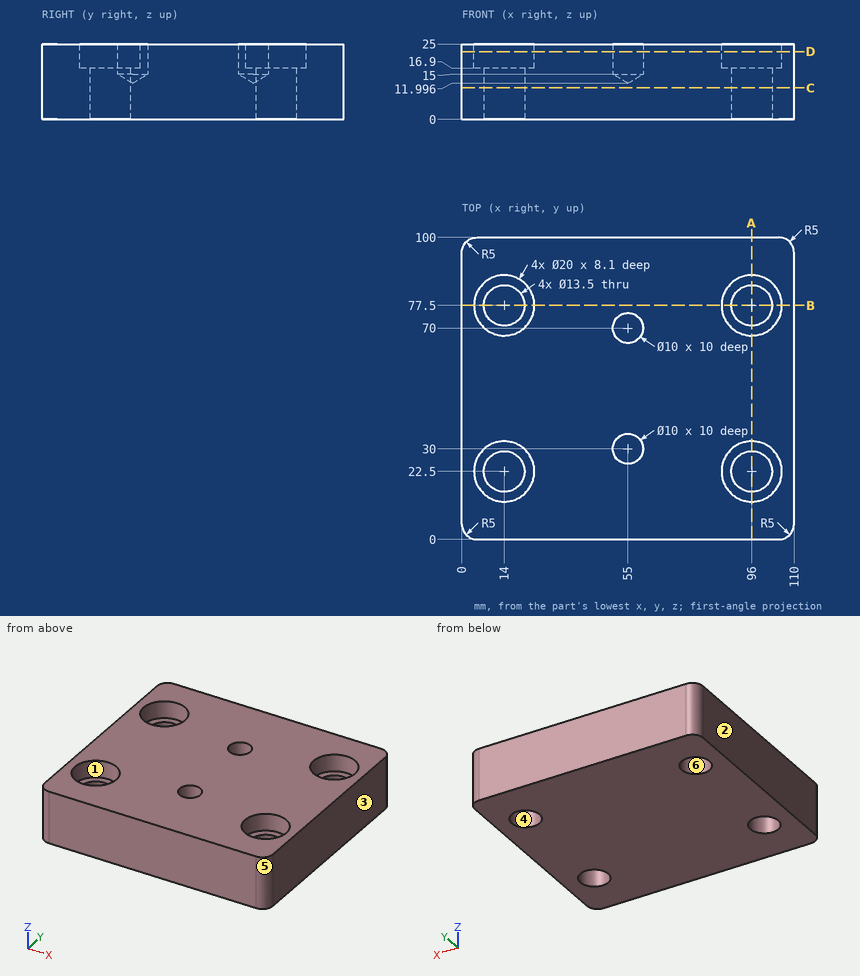
Part print with two shaded views. Sizes in mm from the minimum x, y, z corner. A direction names the side the tool comes from. Round coordinates to 2 decimals unless told otherwise and drop trailing zeros. Loops run counter-clockwise (first coordinate to the right, second up) from the corner with the lowest first, then second, coordinate; pieces in that order, holes last.
1. Slice it at B-B (y = 77.5). Give the cut face in (x, z), and give its area (3 significant figures).
Solutions:
outline: (0, 0) - (7.25, 0) - (7.25, 16.9) - (4, 16.9) - (4, 25) - (0, 25) - close; (20.75, 0) - (89.25, 0) - (89.25, 16.9) - (86, 16.9) - (86, 25) - (24, 25) - (24, 16.9) - (20.75, 16.9) - close; (102.75, 0) - (110, 0) - (110, 25) - (106, 25) - (106, 16.9) - (102.75, 16.9) - close
area: 1,970 mm2
2. Slice it at C-C (z = 10.5). Give the cut face in (x, y).
Solutions:
outline: (0, 5) arc R5 ccw to (5, 0) - (105, 0) arc R5 ccw to (110, 5) - (110, 95) arc R5 ccw to (105, 100) - (5, 100) arc R5 ccw to (0, 95) - close; hole circle Ø13.5 at (14, 22.5); hole circle Ø13.5 at (14, 77.5); hole circle Ø13.5 at (96, 22.5); hole circle Ø13.5 at (96, 77.5)
3. Drill centre lines: line 1 along Y through (x, z) = (14, 22.25); line 2 along Y through (x, z) = (14, 9.5); line 3 along X through (y, z) = (17.5, 6.5) (1 decimal). Where is each one in solid material? Low to high.
Solutions:
line 1: y = 0 to 12.5, 32.5 to 67.5, 87.5 to 100
line 2: y = 0 to 15.75, 29.25 to 70.75, 84.25 to 100
line 3: x = 0 to 9.5, 18.5 to 91.5, 100.5 to 110
4. Slice it at A-A (x = 96). Give the cut face in (y, z).
Solutions:
outline: (0, 0) - (15.75, 0) - (15.75, 16.9) - (12.5, 16.9) - (12.5, 25) - (0, 25) - close; (29.25, 0) - (70.75, 0) - (70.75, 16.9) - (67.5, 16.9) - (67.5, 25) - (32.5, 25) - (32.5, 16.9) - (29.25, 16.9) - close; (84.25, 0) - (100, 0) - (100, 25) - (87.5, 25) - (87.5, 16.9) - (84.25, 16.9) - close
5. Two-plate mould, pull along Y, no slides. Class the marked faces 3, 4, 5 and 6: pulls with the +Y half, pulls with the -Y half, needs draft (parallel to the pull), parting line crosses it, or undercut.
Solutions:
face 3: needs draft
face 4: undercut
face 5: pulls with the -Y half
face 6: undercut
6. Slice it at D-D (z = 22.5). Give the cut face in (x, y).
Solutions:
outline: (0, 5) arc R5 ccw to (5, 0) - (105, 0) arc R5 ccw to (110, 5) - (110, 95) arc R5 ccw to (105, 100) - (5, 100) arc R5 ccw to (0, 95) - close; hole circle Ø20 at (14, 22.5); hole circle Ø20 at (14, 77.5); hole circle Ø10 at (55, 30); hole circle Ø10 at (55, 70); hole circle Ø20 at (96, 22.5); hole circle Ø20 at (96, 77.5)
7. Flat gauge pins, fed straight in: pin 1 (18 mm diameter, centred on x = 14, y = 77.5, fed in from +Z); pin 2 (23 mm diameter, centred on x = 14, y = 22.5, fed in from +Z). Where does each tip first touch, or does it go through?
Solutions:
pin 1: stops at z = 16.9
pin 2: stops at z = 25
8. 3-axis set-ups, long thin cutter, end or side, ignore diameter. For the marked faces 1 and 2: which of +Z, -Z, +X, -X, +Y, -Y reach the whole face in a straight line?
Solutions:
face 1: +Z
face 2: +Z, -Z, -X, +Y, -Y
